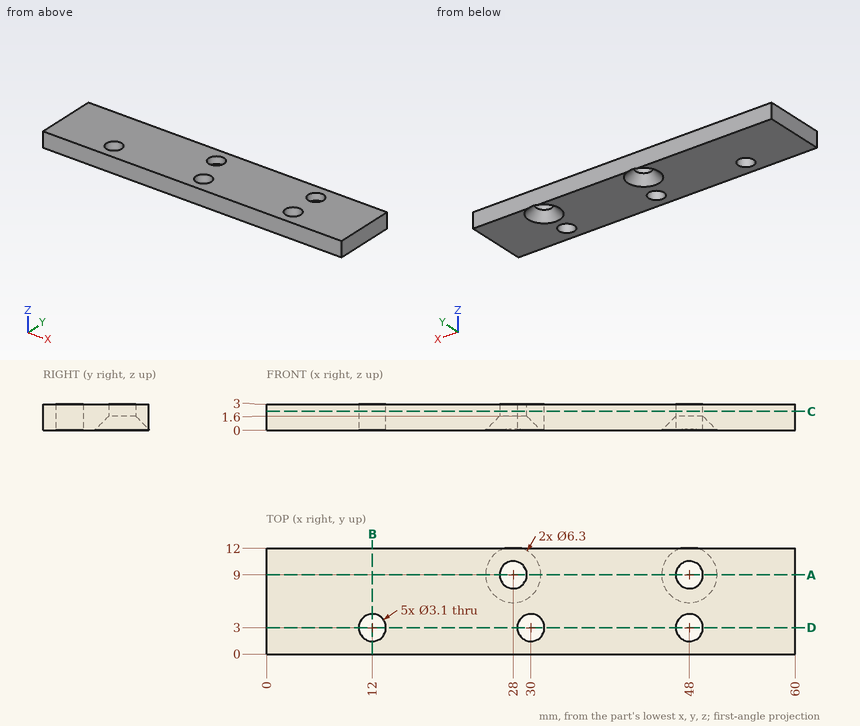
The figure shows three views and two pictorial views of one solid part (mm, origin at its lowest corner). Answer the questions. Give positions to 0.01 mm unless a question says otherwise; leave off trailing zeros. Write each loop counter-clockwise with the first axis right and the second up, starting at its lowest first coordinate (ties: lowest second). Pieces come first, ordered by that corner, then holes. Notation, with made-up numbers: (29.5, -20.75) - (72.5, -20.75) arc R26 cw to (72.5, 4.25) - close; hole circle Ø7 at (43, -16). An arc over 180 degrees is marked (long way). Use one line per item in the form item = value.
1. A cutting plane is placed at A-A (y = 9). Write down the section's boundary in (x, z).
Filled in:
outline = (0, 0) - (24.85, 0) - (26.45, 1.6) - (26.45, 3) - (0, 3) - close; (29.55, 1.6) - (31.15, 0) - (44.85, 0) - (46.45, 1.6) - (46.45, 3) - (29.55, 3) - close; (49.55, 1.6) - (51.15, 0) - (60, 0) - (60, 3) - (49.55, 3) - close
2. A cutting plane is placed at B-B (x = 12). Write down the section's boundary in (y, z).
Filled in:
outline = (0, 0) - (1.45, 0) - (1.45, 3) - (0, 3) - close; (4.55, 0) - (12, 0) - (12, 3) - (4.55, 3) - close
3. A cutting plane is placed at C-C (z = 2.15). Write down the section's boundary in (x, y).
Filled in:
outline = (0, 0) - (60, 0) - (60, 12) - (0, 12) - close; hole circle Ø3.1 at (12, 3); hole circle Ø3.1 at (28, 9); hole circle Ø3.1 at (30, 3); hole circle Ø3.1 at (48, 3); hole circle Ø3.1 at (48, 9)
4. A cutting plane is placed at D-D (y = 3). Write down the section's boundary in (x, z), and give its area (3 significant figures).
Filled in:
outline = (0, 0) - (10.45, 0) - (10.45, 3) - (0, 3) - close; (13.55, 0) - (28.45, 0) - (28.45, 3) - (13.55, 3) - close; (31.55, 0) - (46.45, 0) - (46.45, 3) - (31.55, 3) - close; (49.55, 0) - (60, 0) - (60, 3) - (49.55, 3) - close
area = 152 mm^2
5. Consider L1, parallel to X at y = 9.5, z = 2.75; L2, parallel to X at y = 4.25, z = 2.65; L3, parallel to Y at x = 12, z = 2.35. Determine where each line is inside the solid, lowest interval first.
Filled in:
L1 = 0 to 26.53, 29.47 to 46.53, 49.47 to 60
L2 = 0 to 11.08, 12.92 to 29.08, 30.92 to 47.08, 48.92 to 60
L3 = 0 to 1.45, 4.55 to 12
